```python
from build123d import *

# Parameters (mm, degrees)
SKETCH_R     = 14.5
SKETCH001_R  = 11.5
SKETCH003_R  = 10.5
SKETCH002_R  = 13.5
SKETCH004_R  = 11.547972
PAD_DEPTH    = 1
SKETCH005_R  = 2.5
POCKET_DEPTH = 5


with BuildPart() as part:
    # Sketch → AdditiveLoft section 0
    with BuildSketch(Plane.XZ):
        Circle(SKETCH_R)
    # Sketch001 (on DatumPlane) → AdditiveLoft section 1
    with BuildSketch(Plane.XZ.offset(-4)):
        with Locations((0, -0.047972)):
            Circle(SKETCH001_R)
    loft()

    # Sketch003 (on Face3 of AdditiveLoft) → SubtractiveLoft section 0
    with BuildSketch(Plane(origin=(0, 4, 0), x_dir=(1, 0, 0), z_dir=(0, 1, 0))):
        Circle(SKETCH003_R)
    # Sketch002 (on Face1 of AdditiveLoft) → SubtractiveLoft section 1
    with BuildSketch(Plane.XZ):
        Circle(SKETCH002_R)
    loft(mode=Mode.SUBTRACT)

    # Sketch004 (on Face4 of SubtractiveLoft) → Pad (new body)
    with BuildSketch(Plane(origin=(0, 4, 0), x_dir=(1, 0, 0), z_dir=(0, 1, 0))):
        Circle(SKETCH004_R)
    extrude(amount=-PAD_DEPTH)

    # Sketch005 (on Face9 of Pad) → Pocket (cut)
    with BuildSketch(Plane(origin=(0, 4, 0), x_dir=(1, 0, 0), z_dir=(0, 1, 0))):
        Circle(SKETCH005_R)
    extrude(amount=-POCKET_DEPTH, mode=Mode.SUBTRACT)


solid = part.part
```
Input: part model. Units: mm. Frame: model coordinates. Coordinates: 2 decimals unless noted, no trailing zeros. Use a Markdown table: item, result.
1) Material intervals for line 1 along Y through (x, z) = (-4, 1.5); line 2 along X through (y, z) = (3.45, 0); line 3 along X through (y, z) = (0.65, -3), sorted ascending. Write a range as from..to.
Results found:
| item | result |
|---|---|
| line 1 | y = 3..4 |
| line 2 | x = -11.91..-2.5, 2.5..11.91 |
| line 3 | x = -13.69..-12.66, 12.66..13.69 |
2) Pull-direction query (X, two-part tool) for faces 1 (the flat face through (-3, 4, 0)), 2 (the conical face through (-2.47, 2.81, 11.12)), 3 (the flat face through (0, 3, -3)); classes: released by +X, released by -X, zero draft, split by the parting line, or undercut.
Results found:
| item | result |
|---|---|
| face 1 | zero draft |
| face 2 | undercut |
| face 3 | undercut |
3) Contact query for flat-ended pins moving along their axis: pin 1 (3 mm diameter, centred on x = -1, z = 1.5, fed in from -Y); pin 2 (8 mm diameter, centred on x = 0, z = 0, fed in from +Y). Output: stop coordinate, or through.
Results found:
| item | result |
|---|---|
| pin 1 | stops at y = 3 |
| pin 2 | stops at y = 4 |
